```python
from build123d import *

# Parameters (mm, degrees)
BOSS_EXTRUDE1_START      = -1
SKETCH1_W                = 1.7
SKETCH1_H                = 89.2
BOSS_EXTRUDE1_DEPTH      = 8.8
SKETCH4_W                = 33.7
SKETCH4_H                = 11.6
BOSS_EXTRUDE3_DEPTH      = 8.8
SERVO_HOLDER_DEPTH       = 1
SERVO_HOLDER_DEPTH_BACK  = 8.8
SKETCH3_W                = 14
SKETCH3_H                = 7
SKETCH3_R                = 1
SKETCH37_W               = 20
SKETCH37_H               = 7
BOSS_EXTRUDE19_DEPTH     = 9.8
CUT_EXTRUDE10_DEPTH      = 93.434679639
CUT_EXTRUDE10_DEPTH_BACK = 93.434679639
SKETCH29_W               = 34.409909993
SKETCH29_H               = 6.377389624
BOSS_EXTRUDE13_START     = 2
SKETCH30_W               = 34
SKETCH30_H               = 38
SKETCH30_R               = 1.6
BOSS_EXTRUDE13_DEPTH     = 6.5
SKETCH41_W               = 17.288461538
SKETCH41_H               = 8.8
CUT_EXTRUDE14_DEPTH      = 15
BOSS_EXTRUDE14_START     = -38
SKETCH32_R               = 1.45
SKETCH32_R_2             = 5.2
BOSS_EXTRUDE14_DEPTH     = 8.8
BOSS_EXTRUDE16_DEPTH     = 3
BOSS_EXTRUDE17_DEPTH     = 3
BOSS_EXTRUDE18_DEPTH     = 8.8
SKETCH39_W               = 1.7
SKETCH39_H               = 41.2
BOSS_EXTRUDE20_DEPTH     = 8.8
CUT_EXTRUDE13_DEPTH      = 17.5
CHAMFER2_SIZE            = 0.6
CHAMFER2_SIZE_2          = 1.039230485
CHAMFER3_SIZE            = 3
FILLET10_R               = 6
CUT_EXTRUDE15_DEPTH      = 10
CHAMFER4_SIZE            = 2.5
CUT_EXTRUDE16_DEPTH      = 10
FILLET11_R               = 0.8
SKETCH44_W               = 34
SKETCH44_H               = 48.2
SKETCH44_W_2             = 31.2
SKETCH44_H_2             = 45.4
BOSS_EXTRUDE21_DEPTH     = 100


with BuildPart() as part:
    # Sketch1 → Boss-Extrude1 (new body)
    with BuildSketch(Plane(origin=(0, 0, 0), x_dir=(1, 0, 0), z_dir=(0, 1, 0)).offset(BOSS_EXTRUDE1_START)):
        with Locations((-20.85, 25.311538462)):
            Rectangle(SKETCH1_W, SKETCH1_H)
    extrude(amount=-BOSS_EXTRUDE1_DEPTH)

    # Sketch4 → Boss-Extrude3 (add)
    with BuildSketch(Plane.XZ.offset(9.8)):
        with Locations((-4.85, -64.111538462)):
            Rectangle(SKETCH4_W, SKETCH4_H)
    extrude(amount=-BOSS_EXTRUDE3_DEPTH)

    # Sketch3 → Servo Holder (add, two sides: drawn at the far end of the back side and taken through both)
    # profile 1 of 2: a face of its own
    with BuildSketch(Plane.XZ.offset(9.8).offset(-SERVO_HOLDER_DEPTH_BACK)):
        with Locations((-14.7, -55.411538462)):
            Rectangle(SKETCH3_W, SKETCH3_H)
        with Locations(Location((-14, -54.311538462, 0), (0, 0, 270))):
            Circle(SKETCH3_R, mode=Mode.SUBTRACT)
    # profile 2 of 2: a face of its own
    with BuildSketch(Plane.XZ.offset(9.8).offset(-SERVO_HOLDER_DEPTH_BACK)):
        with Locations((-14.7, -25.211538462)):
            Rectangle(SKETCH3_W, SKETCH3_H)
        with Locations(Location((-14, -26.311538462, 0), (0, 0, 90))):
            Circle(SKETCH3_R, mode=Mode.SUBTRACT)
    extrude(amount=SERVO_HOLDER_DEPTH + SERVO_HOLDER_DEPTH_BACK)

    # Sketch37 → Boss-Extrude19 (add)
    with BuildSketch(Plane(origin=(0, -1, 0), x_dir=(1, 0, 0), z_dir=(0, 1, 0))):
        with Locations((2.3, 25.211538462)):
            Rectangle(SKETCH37_W, SKETCH37_H)
    extrude(amount=-BOSS_EXTRUDE19_DEPTH)

    # Sketch29 → Cut-Extrude10 (cut, two sides: drawn at the far end of the back side and taken through both)
    with BuildSketch(Plane(origin=(0, 0, -69.911538462), x_dir=(-1, 0, 0), z_dir=(0, 0, -1)).offset(-CUT_EXTRUDE10_DEPTH_BACK)):
        with Locations((4.495045004, -12.988694812)):
            Rectangle(SKETCH29_W, SKETCH29_H)
    extrude(amount=CUT_EXTRUDE10_DEPTH + CUT_EXTRUDE10_DEPTH_BACK, mode=Mode.SUBTRACT)


with BuildPart() as body_2:
    # Sketch30 → Boss-Extrude13 (new body)
    with BuildSketch(Plane.XY.offset(BOSS_EXTRUDE13_START)):
        with Locations((-4.7, -20)):
            Rectangle(SKETCH30_W, SKETCH30_H)
        with Locations(Location((5.3, -34, 0), (0, 0, 180))):
            Circle(SKETCH30_R, mode=Mode.SUBTRACT)
        with Locations(Location((5.3, -19, 0), (0, 0, 180))):
            Circle(SKETCH30_R, mode=Mode.SUBTRACT)
        with Locations(Location((-14.7, -34, 0), (0, 0, 180))):
            Circle(SKETCH30_R, mode=Mode.SUBTRACT)
        with Locations(Location((-14.7, -19, 0), (0, 0, 180))):
            Circle(SKETCH30_R, mode=Mode.SUBTRACT)
    extrude(amount=BOSS_EXTRUDE13_DEPTH)


with BuildPart() as cut_extrude14_tool:
    # Sketch41 → Cut-Extrude14 (new body)
    with BuildSketch(Plane(origin=(-20, 0, 0), x_dir=(0, 0, -1), z_dir=(1, 0, 0))):
        with Locations((-10.644230769, -5.4)):
            Rectangle(SKETCH41_W, SKETCH41_H)
    extrude(amount=-CUT_EXTRUDE14_DEPTH)


with BuildPart() as part_1:
    add(part.part)

    # Cut-Extrude14: cut by cut_extrude14_tool
    add(cut_extrude14_tool.part, mode=Mode.SUBTRACT)



with BuildPart() as body_2_1:
    add(body_2.part)

    # Cut-Extrude14: cut by cut_extrude14_tool
    add(cut_extrude14_tool.part, mode=Mode.SUBTRACT)

    # Sketch32 → Boss-Extrude14 (add)
    with BuildSketch(Plane.XZ.offset(39).offset(BOSS_EXTRUDE14_START)):
        with BuildLine():
            ThreePointArc((11.872921748, 2), (25.925390485, -3.535644523), (35.05, 8.5))
            ThreePointArc((35.05, 8.5), (22.55, 21), (10.05, 8.5))
            Line((10.05, 8.5), (12.3, 8.5))
            Line((12.3, 8.5), (12.3, 2))
            Line((12.3, 2), (11.872921748, 2))
        make_face()
        with Locations(Location((16.410078628, 3.371514303, 0), (0, 0, 180))):
            Circle(SKETCH32_R, mode=Mode.SUBTRACT)
        with Locations(Location((27.678485697, 2.360078628, 0), (0, 0, 180))):
            Circle(SKETCH32_R, mode=Mode.SUBTRACT)
        with Locations(Location((17.421514303, 14.639921372, 0), (0, 0, 180))):
            Circle(SKETCH32_R, mode=Mode.SUBTRACT)
        with Locations(Location((22.55, 8.5, 0), (0, 0, 180))):
            Circle(SKETCH32_R_2, mode=Mode.SUBTRACT)
        with Locations(Location((28.689921372, 13.628485697, 0), (0, 0, 180))):
            Circle(SKETCH32_R, mode=Mode.SUBTRACT)
    extrude(amount=BOSS_EXTRUDE14_DEPTH)


with BuildPart() as part_2:
    add(part_1.part)

    add(body_2_1.part)  # Boss-Extrude16 merges body 2
    # Sketch34 → Boss-Extrude16 (add)
    with BuildSketch(Plane.ZY.offset(21.7)):
        Polygon((-21.711538462, -1), (-21.711538462, -9.8), (2, -39), (8.5, -39), (8.5, -1), align=None)
    extrude(amount=-BOSS_EXTRUDE16_DEPTH)

    # Sketch35 → Boss-Extrude17 (add)
    with BuildSketch(Plane(origin=(12.3, 0, 0), x_dir=(0, 0, -1), z_dir=(1, 0, 0))):
        Polygon((-2, -1), (21.711538462, -1), (21.711538462, -9.8), (-2, -39), (-8.5, -39), (-8.5, -9.8), (-8.5, -1), align=None)
    extrude(amount=-BOSS_EXTRUDE17_DEPTH)

    # Sketch36 → Boss-Extrude18 (add)
    with BuildSketch(Plane.XZ.offset(9.8)):
        Polygon((12.3, -10.579162849), (16.63422252, -2.511520186), (12.3, 1.345455989), align=None)
    extrude(amount=-BOSS_EXTRUDE18_DEPTH)

    # Sketch39 → Boss-Extrude20 (add)
    with BuildSketch(Plane(origin=(0, -1, 0), x_dir=(1, 0, 0), z_dir=(0, 1, 0))):
        with Locations((11.45, 49.311538462)):
            Rectangle(SKETCH39_W, SKETCH39_H)
    extrude(amount=-BOSS_EXTRUDE20_DEPTH)

    # Sketch40 → Cut-Extrude13 (cut)
    with BuildSketch(Plane(origin=(12.3, 0, 0), x_dir=(0, 0, -1), z_dir=(1, 0, 0))):
        Polygon((64.111538462, -1), (60.611538462, -1), (60.611538462, -2.2), (59.611538462, -2.2), (59.611538462, -6.2), (64.111538462, -6.2), align=None)
        Polygon((67.611538462, -1), (64.111538462, -1), (64.111538462, -6.2), (68.611538462, -6.2), (68.611538462, -2.2), (67.611538462, -2.2), align=None)
    extrude(amount=-CUT_EXTRUDE13_DEPTH, mode=Mode.SUBTRACT)

    # Chamfer2
    # the kernel refuses this chamfer: 1.039230485, 0.6 mm, written as the material it takes off along each edge
    with BuildSketch(Plane(origin=(14.988578382, -2.2, -67.611538462), x_dir=(0, 0.9983227437537925, 0.05789386240267319), z_dir=(-1, 0, 0))) as chamfer2_piece_1_section:
        Polygon((CHAMFER2_SIZE * 0.998322743754, CHAMFER2_SIZE * 0.0578938624027), (-CHAMFER2_SIZE_2 * 0.0578938623771, CHAMFER2_SIZE_2 * 0.998322743313), (0, 0), align=None)
    chamfer2_piece_1 = extrude(amount=20.188578382, mode=Mode.PRIVATE)
    chamfer2_piece_1 = split(chamfer2_piece_1, bisect_by=Plane(origin=(4.894289191, -2.005782009, -68.611538462), z_dir=(0, 0, 1)), keep=Keep.TOP, mode=Mode.PRIVATE)
    add(chamfer2_piece_1, mode=Mode.SUBTRACT)
    with BuildSketch(Plane(origin=(14.988578382, -2.2, -60.611538462), x_dir=(0, 0.9983227437537925, -0.05789386240267317), z_dir=(-1, 0, 0))) as chamfer2_piece_2_section:
        Polygon((CHAMFER2_SIZE * 0.998322743754, -CHAMFER2_SIZE * 0.0578938624027), (-CHAMFER2_SIZE_2 * 0.0578938623771, -CHAMFER2_SIZE_2 * 0.998322743313), (0, 0), align=None)
    chamfer2_piece_2 = extrude(amount=20.188578382, mode=Mode.PRIVATE)
    chamfer2_piece_2 = split(chamfer2_piece_2, bisect_by=Plane(origin=(4.894289191, -2.005782009, -59.611538462), z_dir=(0, 0, -1)), keep=Keep.TOP, mode=Mode.PRIVATE)
    add(chamfer2_piece_2, mode=Mode.SUBTRACT)

    # Chamfer3
    chamfer3_edges = [part_2.edges().sort_by_distance(p)[0] for p in [
        (10.6, -5.4, -58.311538462),
        (10.6, -5.4, -28.711538462),
    ]]
    chamfer(chamfer3_edges, length=CHAMFER3_SIZE)

    # Fillet10
    fillet10_edges = [part_2.edges().sort_by_distance(p)[0] for p in [
        (16.63422252, -5.4, -2.511520186),
        (12.3, -5.4, -10.579162849),
    ]]
    fillet(fillet10_edges, radius=FILLET10_R)

    # Sketch42 → Cut-Extrude15 (cut)
    with BuildSketch(Plane.XY.offset(8.5)):
        with BuildLine():
            Line((-1.1, -1), (-1.1, -10.6))
            ThreePointArc((-1.1, -10.6), (-4.7, -14.2), (-8.3, -10.6))
            Line((-8.3, -10.6), (-8.3, -1))
            Line((-8.3, -1), (-1.1, -1))
        make_face()
    extrude(amount=-CUT_EXTRUDE15_DEPTH, mode=Mode.SUBTRACT)

    # Chamfer4
    chamfer4_edges = [part_2.edges().sort_by_distance(p)[0] for p in [
        (-7.7, -5.4, -58.311538462),
    ]]
    chamfer(chamfer4_edges, length=CHAMFER4_SIZE)

    # Sketch43 → Cut-Extrude16 (cut)
    with BuildSketch(Plane(origin=(0, -1, 0), x_dir=(1, 0, 0), z_dir=(0, 1, 0))):
        Polygon((-5.2, 58.311538462), (-11.6, 51.911538462), (-5.2, 51.911538462), align=None)
    extrude(amount=-CUT_EXTRUDE16_DEPTH, mode=Mode.SUBTRACT)

    # Fillet11
    fillet11_edges = [part_2.edges().sort_by_distance(p)[0] for p in [
        (-20, -5.4, -28.711538462),
        (-20, -5.4, -51.911538462),
        (10.6, -5.4, -55.311538462),
        (10.6, -5.4, -31.711538462),
        (7.6, -5.4, -28.711538462),
        (7.6, -5.4, -58.311538462),
        (-5.2, -5.4, -58.311538462),
        (-11.6, -5.4, -51.911538462),
    ]]
    fillet(fillet11_edges, radius=FILLET11_R)

    # Sketch44 → Boss-Extrude21 (add)
    with BuildSketch(Plane(origin=(0, -9.8, 0), x_dir=(-1, 0, 0), z_dir=(0, -1, 0))):
        with Locations((4.7, 45.811538462)):
            Rectangle(SKETCH44_W, SKETCH44_H)
        with Locations((4.7, 45.811538462)):
            Rectangle(SKETCH44_W_2, SKETCH44_H_2, mode=Mode.SUBTRACT)
    extrude(amount=BOSS_EXTRUDE21_DEPTH)


solid = part_2.part
```
For this review, take the finished solid that the model builds, in its own axes (mm). A direction names the side the tool comes from. Round coordinates to 2 decimals unless told otherwise and drop trailing zeros. Write each loop counter-clockwise with the first axis right and the second up, starting at its lowest first coordinate (ties: lowest second). Pieces come first, ordered by that corner, then holes. Notation, with made-up numbers: (4, 84.25) - (9, 84.25) arc R17 ccw to (9, 92.25) - close; hole circle Ø11 at (3.25, 60). An arc over 180 degrees is marked (long way). Put each result on its own line as item: value.
Q1. We need section A-A (y = -19). Give the boundary of the cut face in (x, z).
Solved:
outline: (-21.7, -69.91) - (12.3, -69.91) - (12.3, -21.71) - (-21.7, -21.71) - close; (-21.7, -14.24) - (-18.7, -14.24) - (-18.7, 2) - (-16.3, 2) - (-16.3, 8.5) - (-21.7, 8.5) - close; (-13.1, 2) - (3.7, 2) - (3.7, 8.5) - (-13.1, 8.5) - close; (6.9, 2) - (9.3, 2) - (9.3, -14.24) - (12.3, -14.24) - (12.3, 8.5) - (6.9, 8.5) - close; hole (-20.3, -68.51) - (10.9, -68.51) - (10.9, -23.11) - (-20.3, -23.11) - close
Q2. Machinability: for faces 4 (the face through (-20.3, -59, -45)), 5 (the face through (9.3, -16, -7)), 6 (the face through (-5, -39, 5)), 7 (the face through (-15.56, -20.35, 5.2)), which of the approach directions +Z, -Z, +X, -X, +Y, -Y give a long, thin tool a straight path to every point of the face, cutting with its end or side? Answer none if there is none.
Solved:
face 4: -Y
face 5: +Y, -Y
face 6: +Z, +X, -X, -Y
face 7: +Z
Q3. We need section B-B (x = 22.55). Give the boundary of the cut face in (y, z).
Solved:
outline: (-9.8, -4) - (-1, -4) - (-1, 3.3) - (-9.8, 3.3) - close; (-9.8, 13.7) - (-1, 13.7) - (-1, 21) - (-9.8, 21) - close
Q4. Wall thickness on probe 1 along Z at (x, y) = (-11, -14); probe 2 along X at (y, z) = (-19, 5.5); probe 3 along X at (y, z) = (-6, 8): over which ranges is each line inside the solid? List them lowest first.
Solved:
probe 1: z = -69.91 to -68.51, -23.11 to -21.71, 2 to 8.5
probe 2: x = -21.7 to -16.3, -13.1 to 3.7, 6.9 to 12.3
probe 3: x = -21.7 to -8.3, -1.1 to 17.37, 27.73 to 35.04
Q5. Mouldability with a two-part tool opening along Z and no side actions: class faces 1 (the face through (-4, -55, -69.912)), 2 (the face through (-4.6, -14.2, 5.3)), 3 (the face through (1, -5, -58.312)) as released by +Z, released by -Z, zero draft, split by the parting line, or undercut.
Solved:
face 1: released by -Z
face 2: zero draft
face 3: undercut
Q6. We need section D-D (y = -86). Give the boundary of the cut face in (x, z).
Solved:
outline: (-21.7, -69.91) - (12.3, -69.91) - (12.3, -21.71) - (-21.7, -21.71) - close; hole (-20.3, -68.51) - (10.9, -68.51) - (10.9, -23.11) - (-20.3, -23.11) - close
Q7. Insertion check: pin 1 Ø17 at (x, y) = (-7, -24) entering from +Z; pin 2 Ø4 at (y, z) = (-2.5, -64) entering from +X; pin 3 Ø4 at (x, z) = (26.5, -1) entering from -Y. Each pin has a flat end and moves straight along its axis. Give the tip position at first contact, or say it passes through.
Solved:
pin 1: stops at z = 8.5
pin 2: stops at x = -5.2
pin 3: stops at y = -9.8
Q8. We need section C-C (z = -40). Give the boundary of the cut face in (x, y), and give its area (3 significant figures).
Solved:
outline: (-21.7, -109.8) - (-20.3, -109.8) - (-20.3, -9.8) - (-20, -9.8) - (-20, -1) - (-21.7, -1) - close; (10.6, -9.8) - (10.9, -9.8) - (10.9, -109.8) - (12.3, -109.8) - (12.3, -1) - (10.6, -1) - close
area: 310 mm2
